```python
from build123d import *

# Parameters (mm, degrees)
BOSS_EXTRUDE1_DEPTH      = 254
BOSS_EXTRUDE1_DEPTH_BACK = 185.42
SKETCH1_W                = 12.7
SKETCH1_H                = 12.7
SKETCH1_W_2              = 9.525
SKETCH1_H_2              = 9.525
CUT_EXTRUDE1_DEPTH       = 255.158700422
CUT_EXTRUDE1_DEPTH_BACK  = 255.158700422
SKETCH4_R                = 3.96875
CUT_EXTRUDE3_DEPTH       = 255.396565425
SKETCH5_W                = 3.175
SKETCH5_H                = 13.97
CUT_EXTRUDE4_DEPTH       = 440.511753426


with BuildPart() as part:
    # Sketch1 → Boss-Extrude1 (new, two sides: drawn at the far end of the back side and taken through both)
    with BuildSketch(Plane(origin=(0, 0, 0), x_dir=(0, 0, -1), z_dir=(1, 0, 0)).offset(-BOSS_EXTRUDE1_DEPTH_BACK)):
        Rectangle(SKETCH1_W, SKETCH1_H)
        Rectangle(SKETCH1_W_2, SKETCH1_H_2, mode=Mode.SUBTRACT)
    extrude(amount=BOSS_EXTRUDE1_DEPTH + BOSS_EXTRUDE1_DEPTH_BACK)

    # Sketch2 → Cut-Extrude1 (cut, two sides: drawn at the far end of the back side and taken through both)
    with BuildSketch(Plane(origin=(0, 0, 0), x_dir=(1, 0, 0), z_dir=(0, 1, 0)).offset(-CUT_EXTRUDE1_DEPTH_BACK)):
        Polygon((-185.42, -6.35), (-174.250456919, 6.961343094), (-183.078216502, 14.368712905), (-194.247759583, 1.057369811), align=None)
    extrude(amount=CUT_EXTRUDE1_DEPTH + CUT_EXTRUDE1_DEPTH_BACK, mode=Mode.SUBTRACT)

    # Sketch4 → Cut-Extrude3 (cut, through all)
    with BuildSketch(Plane.XY.offset(6.35)):
        with Locations((241.3, 0)):
            Circle(SKETCH4_R)
        with Locations((228.6, 0)):
            Circle(SKETCH4_R)
        with Locations((215.9, 0)):
            Circle(SKETCH4_R)
        with Locations((203.2, 0)):
            Circle(SKETCH4_R)
        with Locations((190.5, 0)):
            Circle(SKETCH4_R)
        with Locations((177.8, 0)):
            Circle(SKETCH4_R)
        with Locations((165.1, 0)):
            Circle(SKETCH4_R)
        with Locations((152.4, 0)):
            Circle(SKETCH4_R)
        with Locations((139.7, 0)):
            Circle(SKETCH4_R)
        with Locations((127, 0)):
            Circle(SKETCH4_R)
        with Locations((114.3, 0)):
            Circle(SKETCH4_R)
        with Locations((101.6, 0)):
            Circle(SKETCH4_R)
        with Locations((88.9, 0)):
            Circle(SKETCH4_R)
        with Locations((76.2, 0)):
            Circle(SKETCH4_R)
        with Locations((63.5, 0)):
            Circle(SKETCH4_R)
        with Locations((50.8, 0)):
            Circle(SKETCH4_R)
        with Locations((38.1, 0)):
            Circle(SKETCH4_R)
        with Locations((25.4, 0)):
            Circle(SKETCH4_R)
        with Locations((12.7, 0)):
            Circle(SKETCH4_R)
        Circle(SKETCH4_R)
        with Locations((-12.7, 0)):
            Circle(SKETCH4_R)
        with Locations((-25.4, 0)):
            Circle(SKETCH4_R)
        with Locations((-38.1, 0)):
            Circle(SKETCH4_R)
        with Locations((-50.8, 0)):
            Circle(SKETCH4_R)
        with Locations((-63.5, 0)):
            Circle(SKETCH4_R)
        with Locations((-76.2, 0)):
            Circle(SKETCH4_R)
        with Locations((-88.9, 0)):
            Circle(SKETCH4_R)
        with Locations((-101.6, 0)):
            Circle(SKETCH4_R)
        with Locations((-114.3, 0)):
            Circle(SKETCH4_R)
    extrude(amount=-CUT_EXTRUDE3_DEPTH, mode=Mode.SUBTRACT)

    # Sketch5 → Cut-Extrude4 (cut, through all)
    with BuildSketch(Plane(origin=(254, 0, 0), x_dir=(0, 0, -1), z_dir=(1, 0, 0))):
        with Locations((-4.7625, 0)):
            Rectangle(SKETCH5_W, SKETCH5_H)
    extrude(amount=-CUT_EXTRUDE4_DEPTH, mode=Mode.SUBTRACT)


solid = part.part
```
Source: CAD feature listing. Evaluate the final solid. Frame: model axes, mm. A direction names the side the tool comes from. Coordinates: 2 decimals unless noted, no trailing zeros. Loops run counter-clockwise (first coordinate to the right, second up) from the corner with the lowest first, then second, coordinate; pieces in that order, holes last. Notation, with made-up numbers: M 84,33 L 113,33 A26 ccw 113,61 Z; hole C -38.75,1.25 d1. An arc over 180 degrees is marked long. Use a Markdown table: item, result. Add a question column.
Q1. Access query for faces 5 (the flat face through (33, -4.762, -1)), 6 (the cylindrical face through (199.235, 0.174, -5.545)). Directions: +Z, -Z, +X, -X, +Y, -Y. A direction counts if a zero-diameter tool reaches every point of the face in a straight line with its end or side. Return the directions, or none.
Q2. Section query B-B, the plane z = -3.25. Return loops of the section in (x, y), and give its area (3 significant figures).
Q3. Draft query along Y for faces 1 (the flat face through (37, 4, -6.35)), 2 (the cylindrical face through (168.766, -1.52, -5.545)), 3 (the cylindrical face through (232.266, -1.52, -5.545)), 4 (the flat face through (33, -6.35, -2)). Return one class per face: pulls with the +Y half, pulls with the -Y half, needs draft (parallel to the pull), parting line crosses it, or undercut.
Q4. Material intervals for L1, parallel to Y at x = -15.5, z = -2.5; L2, parallel to Z at x = -44, y = -0.5, sorted ascending.
Q5. Section query C-C, the plane y = 0. State how many separate pieces and enclosed holes the cut face has, and give its area (3 significant figures).
Q6. First-contact query: pin 1 (5 mm diameter, centred on x = 0, y = 0, fed in from +Z); pin 2 (3 mm diameter, centred on x = 147, y = 1, fed in from +Z). Flat tips, straight axial feed; report the tip coordinate or a pass-through.
Result:
| question | item | result |
|---|---|---|
| 1 | face 5 | +Z, +X, -X |
| 1 | face 6 | +Z, -Z |
| 2 | outline | M -177.36,-6.35 L 254,-6.35 L 254,-4.76 L -177.36,-4.76 Z; M -177.36,4.76 L 254,4.76 L 254,6.35 L -177.36,6.35 Z |
| 2 | area | 1,370 mm2 |
| 3 | face 1 | needs draft |
| 3 | face 2 | undercut |
| 3 | face 3 | undercut |
| 3 | face 4 | pulls with the -Y half |
| 4 | L1 | y = -6.35 to -4.76, 4.76 to 6.35 |
| 4 | L2 | z = -6.35 to -4.76 |
| 5 | separate pieces | 30 |
| 5 | enclosed holes | 0 |
| 5 | area | 316 mm2 |
| 6 | pin 1 | passes through |
| 6 | pin 2 | stops at z = -4.76 |
